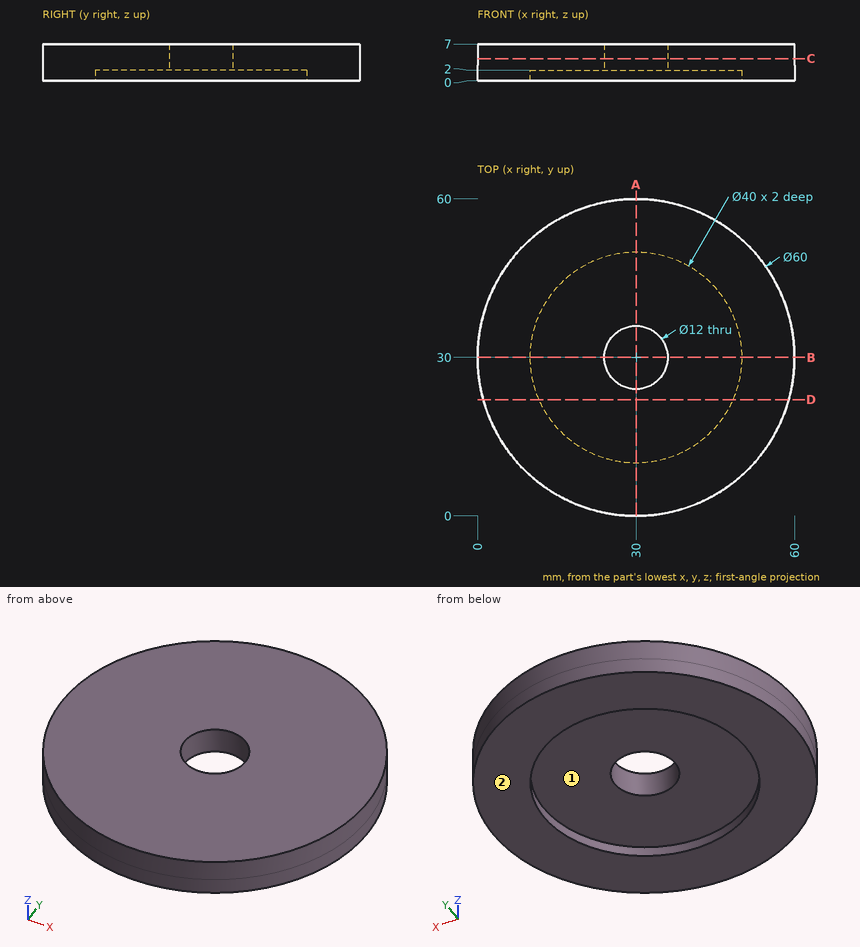
Job drawing, mm, ordinate dimensions from the low corner. One solid piece. Round coordinates to 2 decimals unless told otherwise and drop trailing zeros. Write each loop counter-clockwise with the first axis right and the second up, starting at its lowest first coordinate (ties: lowest second). Pieces come first, ordered by that corner, then holes. Notation, with made-up numbers: M -12,36.5 L 23,36.5 A8 ccw 23,43.5 Z; hole C 60.25,41 d1. An arc over 180 degrees is marked long. Return JSON: item names as keys, results as strings. Group by question number.
(1) Drill centre lines: probe 1 along Y at (x, z) = (30, 1.35); probe 2 along Y at (x, z) = (30, 4.2); probe 3 along X at (y, z) = (34, 1.5). Where is each one in solid material? Low to high.
(2) Pin check, flat tips, straight feed: pin 1 Ø11 at (x, y) = (30, 30) entering from +Z; pin 2 Ø2 at (y, z) = (52.5, 4.5) entering from -X; pin 3 Ø12 at (x, y) = (28.5, 32.5) entering from -Z; pin 4 Ø1 at (x, z) = (21.5, 4) entering from +Y. Stop position of each tip, or through.
(3) Saw through at D-D on y = 22. Write the cut outline in (x, z), then the cut area to 3 significant figures.
(4) Two-plate mould, pull along Y, no slides. Class the marked faces 1 and 2: +Y half, -Y half, draft (parallel to the pull), parting line (faces both ways), or undercut.
(5) Saw through at A-A on x = 30. Write the cut outline in (y, z), then the cut area to 3 significant figures.
(6) Saw through at C-C on z = 4.25. Write the cut outline in (x, y), then the cut area to 3 significant figures.
Returned:
{
 "1": {"probe 1": "0 to 10, 50 to 60", "probe 2": "0 to 24, 36 to 60", "probe 3": "0.27 to 10.4, 49.6 to 59.73"},
 "2": {"pin 1": "through", "pin 2": "x = 9.08", "pin 3": "z = 2", "pin 4": "y = 58.91"},
 "3": {"outline": "M 1.09,0 L 11.67,0 L 11.67,2 L 48.33,2 L 48.33,0 L 58.91,0 L 58.91,7 L 1.09,7 Z", "area": "331 mm²"},
 "4": {"face 1": "undercut", "face 2": "draft"},
 "5": {"outline": "M 0,0 L 10,0 L 10,2 L 24,2 L 24,7 L 0,7 Z; M 36,2 L 50,2 L 50,0 L 60,0 L 60,7 L 36,7 Z", "area": "280 mm²"},
 "6": {"outline": "C 30,30 d60; hole C 30,30 d12", "area": "2,710 mm²"}
}
